Build history of the part. All positions in model axes, mm. Coordinates: 2 decimals unless noted, no trailing zeros. Order: outer loops, then holes, each group sorted by start corner. A loop starts at its lowest first (then second) coordinate and runs counter-clockwise, first axis right, second up. Notation, with made-up numbers: (51, 46) - (83, 46) arc R18 ccw to (83, 68) - close; hole circle Ø2 at (-9, -18). An arc over 180 degrees is marked (long way). One line per item, written item: value.
from build123d import *

# Parameters (mm, degrees)
EXTRUDE_1_DEPTH     = 4
EXTRUDE_2_DEPTH     = 4
FILLET_1_R          = 10
CUT_EXTRUDE_1_DEPTH = 142.025706876
SKETCH_4_W          = 6
SKETCH_4_H          = 6
EXTRUDE_7_DEPTH     = 4
SKETCH_6_R          = 1.5
CUT_EXTRUDE_4_DEPTH = 142.774468788


with BuildPart() as part:
    # Эскиз1 → Бобышка-Вытянуть1 (new body)
    with BuildSketch(Plane(origin=(0, 0, 0), x_dir=(1, 0, 0), z_dir=(0, 1, 0))):
        Polygon((-140, -14.5), (-140, 14.5), (-138, 16.5), (-132, 16.5), (-132, 8), (0, 8), (0, -8), (-132, -8), (-132, -16.5), (-138, -16.5), align=None)
    extrude(amount=EXTRUDE_1_DEPTH)

    # Эскиз2 → Бобышка-Вытянуть2 (add)
    # profile 1 of 2: a face of its own
    with BuildSketch(Plane.XZ):
        with BuildLine():
            Line((-63, 16), (-5, 16))
            ThreePointArc((-5, 16), (0, 11), (-5, 6))
            Line((-5, 6), (-63, 6))
            ThreePointArc((-63, 6), (-68, 11), (-63, 16))
        make_face()
        with BuildLine():
            Line((-63, 13), (-5, 13))
            ThreePointArc((-5, 13), (-3, 11), (-5, 9))
            Line((-5, 9), (-63, 9))
            ThreePointArc((-63, 9), (-65, 11), (-63, 13))
        make_face(mode=Mode.SUBTRACT)
    # profile 2 of 2: a face of its own
    with BuildSketch(Plane.XZ):
        with BuildLine():
            Line((-63, -16), (-5, -16))
            ThreePointArc((-5, -16), (0, -11), (-5, -6))
            Line((-5, -6), (-63, -6))
            ThreePointArc((-63, -6), (-68, -11), (-63, -16))
        make_face()
        with BuildLine():
            Line((-63, -13), (-5, -13))
            ThreePointArc((-5, -13), (-3, -11), (-5, -9))
            Line((-5, -9), (-63, -9))
            ThreePointArc((-63, -9), (-65, -11), (-63, -13))
        make_face(mode=Mode.SUBTRACT)
    extrude(amount=-EXTRUDE_2_DEPTH)

    # Скругление1
    # the kernel refuses this fillet: 10 mm, written as the material it adds along each edge
    with BuildSketch(Plane(origin=(-1, 4, 8), x_dir=(1, 0, 0), z_dir=(0, -1, 0))) as fillet_1_piece_1:
        with BuildLine():
            CenterArc((10.90874153, 1.347902551), FILLET_1_R, 173.676623786, 14.069867748)
            Line((0.96958051, 2.44930085), (0.77079729, 2.471328816))
            ThreePointArc((0.77079729, 2.471328816), (0.463030841, 1.233264109), (-0.16, 0.12))
            Line((-0.16, 0.12), (0, -0.2))
            ThreePointArc((0, -0.2), (0.5, -0.2), (0.801825169, -0.026958051))
            Line((0.801825169, -0.026958051), (1, 0))
        make_face()
    extrude(amount=4)
    with BuildSketch(Plane(origin=(-67, 4, 8), x_dir=(-1, 0, 0), z_dir=(0, -1, 0))) as fillet_1_piece_2:
        with BuildLine():
            CenterArc((9.266499161, -10), FILLET_1_R, 90, 62.181860715)
            Line((0.422166387, -5.333333333), (0.245279732, -5.24))
            ThreePointArc((0.245279732, -5.24), (0.785032611, -2.621235013), (-0.16, -0.12))
            Line((-0.16, -0.12), (0, 0.2))
            Line((0, 0.2), (9.266499161, 0.2))
            Line((9.266499161, 0.2), (9.266499161, 0))
        make_face()
    extrude(amount=4)
    with BuildSketch(Plane(origin=(-1, 4, -8), x_dir=(1, 0, 0), z_dir=(0, -1, 0))) as fillet_1_piece_3:
        with BuildLine():
            CenterArc((10.90874153, -1.347902551), FILLET_1_R, 172.253508466, 14.069867748)
            Line((0.96958051, -2.44930085), (0.77079729, -2.471328816))
            ThreePointArc((0.77079729, -2.471328816), (0.463030841, -1.233264109), (-0.16, -0.12))
            Line((-0.16, -0.12), (0, 0.2))
            ThreePointArc((0, 0.2), (0.5, 0.2), (0.801825169, 0.026958051))
            Line((0.801825169, 0.026958051), (1, 0))
        make_face()
    extrude(amount=4)
    with BuildSketch(Plane(origin=(-67, 4, -8), x_dir=(-1, 0, 0), z_dir=(0, -1, 0))) as fillet_1_piece_4:
        with BuildLine():
            CenterArc((9.266499161, 10), FILLET_1_R, 207.818139285, 62.181860715)
            Line((0.422166387, 5.333333333), (0.245279732, 5.24))
            ThreePointArc((0.245279732, 5.24), (0.785032611, 2.621235013), (-0.16, 0.12))
            Line((-0.16, 0.12), (0, -0.2))
            Line((0, -0.2), (9.266499161, -0.2))
            Line((9.266499161, -0.2), (9.266499161, 0))
        make_face()
    extrude(amount=4)

    # Эскиз3 → Вырез-Вытянуть1 (cut, through all)
    with BuildSketch(Plane.XZ):
        with BuildLine():
            Line((-24.447568559, 3.753765504), (-128.9506377, 3.753765504))
            ThreePointArc((-128.9506377, 3.753765504), (-132.7006377, 0.003765504), (-128.9506377, -3.746234496))
            Line((-128.9506377, -3.746234496), (-24.447568559, -3.746234496))
            ThreePointArc((-24.447568559, -3.746234496), (-20.697568559, 0.003765504), (-24.447568559, 3.753765504))
        make_face()
    extrude(amount=-CUT_EXTRUDE_1_DEPTH, mode=Mode.SUBTRACT)

    # Эскиз4 → Бобышка-Вытянуть7 (add)
    with BuildSketch(Plane(origin=(0, 4, 0), x_dir=(1, 0, 0), z_dir=(0, 1, 0))):
        with Locations((-24, -19)):
            Rectangle(SKETCH_4_W, SKETCH_4_H)
    extrude(amount=-EXTRUDE_7_DEPTH)

    # Эскиз6 → Вырез-Вытянуть4 (cut, through all)
    with BuildSketch(Plane(origin=(0, 4, 0), x_dir=(1, 0, 0), z_dir=(0, 1, 0))):
        with Locations(Location((-24, -19, 0), (0, 0, 270))):
            Circle(SKETCH_6_R)
    extrude(amount=-CUT_EXTRUDE_4_DEPTH, mode=Mode.SUBTRACT)


solid = part.part
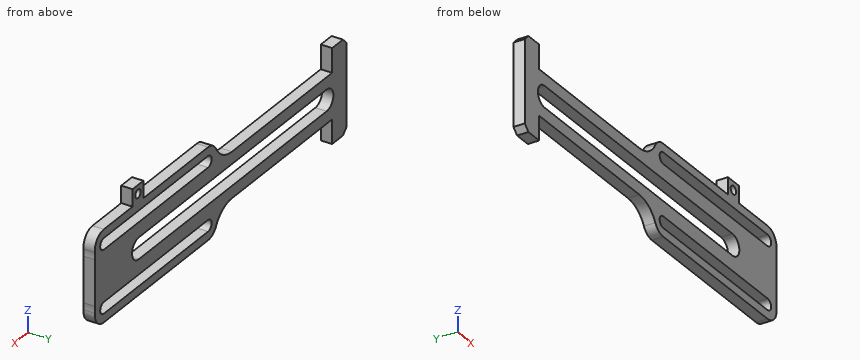
1. Band-saw the part on A-A, the plane z = 19. Give the cut face in (x, y), and give its area (3 significant figures).
Values found:
outline: (-27, 0) - (-25.5, 0) - (-25.5, 4) - (-27, 4) - close; (-22.5, 0) - (-21, 0) - (-21, 4) - (-22.5, 4) - close
area: 12.0 mm2
2. Probe line 1 along Z through (x, y) = (-17, 3.7); line 2 along Z through (x, y) = (-48, 3.7); line 3 along Z through (x, y) = (-81, 3.25). List the from-to ranges inside material, lowest first.
Values found:
line 1: z = -16 to -13, -9 to 9, 13 to 16
line 2: z = -16 to -13, -9 to -3.75, 3.75 to 9, 13 to 16
line 3: z = -8 to -3.75, 3.75 to 8
3. Band-saw the part on C-C, the plane y = 2.3. Count the separate pieces of the cut face and the enclosed holes in it, and give its area (3 significant figures).
Values found:
separate pieces: 1
enclosed holes: 4
area: 2,170 mm2
4. Flat gauge pins, fed straight in: P1, Ø1.2, axis at x = -30, y = 1, coming from the +Z side; P2, Ø2, axis at y = 3, z = 19.5, coming from the +X side; P3, Ø2, axis at x = -111.5, y = 2.5, coming from the +Z side. Where does each tip first touch, or does it go through?
Values found:
P1: stops at z = 16
P2: stops at x = -21
P3: stops at z = 8
5. Band-saw the part on B-B, the plane x = -126.5. Give the cut face in (y, z), and give its area (3 significant figures).
Values found:
outline: (0, -8) - (4, -8) - (4, -3.75) - (0, -3.75) - close; (0, 3.75) - (4, 3.75) - (4, 8) - (0, 8) - close
area: 34.0 mm2
